```python
from build123d import *

# Parameters (mm, degrees)
SKETCH_1_W          = 35
SKETCH_1_H          = 3
EXTRUDE_1_DEPTH     = 3
SKETCH_2_R          = 1.75
CUT_EXTRUDE_1_DEPTH = 10
CHAMFER_1_SIZE      = 2


with BuildPart() as part:
    # Эскиз1 → Бобышка-Вытянуть1 (new body)
    with BuildSketch(Plane.XY):
        Polygon((-32.5, 50), (-32.5, -50), (32.5, -50), (32.5, 50), (17.5, 50), (17.5, 47), (-17.5, 47), (-17.5, 50), align=None)
        with Locations((0, 48.5)):
            Rectangle(SKETCH_1_W, SKETCH_1_H)
        with Locations((0, 51.5)):
            Rectangle(SKETCH_1_W, SKETCH_1_H)
    extrude(amount=EXTRUDE_1_DEPTH)

    # Эскиз2 → Вырез-Вытянуть1 (cut)
    with BuildSketch(Plane.XY.offset(3)):
        with Locations((-25.8, 27.95)):
            Circle(SKETCH_2_R)
        with Locations((-7, 27.95)):
            Circle(SKETCH_2_R)
        with Locations((7, 27.95)):
            Circle(SKETCH_2_R)
        with Locations((25.8, 27.95)):
            Circle(SKETCH_2_R)
        with Locations((-25.8, -27.95)):
            Circle(SKETCH_2_R)
        with Locations((-7, -27.95)):
            Circle(SKETCH_2_R)
        with Locations((7, -27.95)):
            Circle(SKETCH_2_R)
        with Locations((25.8, -27.95)):
            Circle(SKETCH_2_R)
    extrude(amount=-CUT_EXTRUDE_1_DEPTH, mode=Mode.SUBTRACT)

    # Фаска1
    chamfer_1_edges = [part.edges().sort_by_distance(p)[0] for p in [
        (-27.55, -27.95, 0),
        (24.05, 27.95, 0),
        (5.25, 27.95, 0),
        (-8.75, 27.95, 0),
        (-8.75, -27.95, 0),
        (5.25, -27.95, 0),
        (24.05, -27.95, 0),
        (-27.55, 27.95, 0),
    ]]
    chamfer(chamfer_1_edges, length=CHAMFER_1_SIZE)


solid = part.part
```
Design review of the part built by this model. Coordinates are the model's own, in mm. A direction names the side the tool comes from. Round coordinates to 2 decimals unless told otherwise and drop trailing zeros. Order: outer loops, then holes, each group sorted by start corner. A loop starts at its lowest first (then second) coordinate and runs counter-clockwise, first axis right, second up. Notation, with made-up numbers: (11.25, 17) - (32.25, 17) arc R9 cw to (32.25, 22) - close; hole circle Ø7 at (70, 70.5). An arc over 180 degrees is marked (long way). Return JSON: item names as keys, results as strings.
Q1. Consider section C-C on z = 0.55. Give the number of separate pieces and of enclosed holes in the cut face, plus the area to 3 significant figures.
Computed values:
{"separate pieces": "1", "enclosed holes": "8", "area": "6,350 mm2"}
Q2. Consider section D-D on x = -7. Write out the cut boundary in (y, z), plus the area to 3 significant figures.
Computed values:
{"outline": "(-50, 0) - (-31.7, 0) - (-29.7, 2) - (-29.7, 3) - (-50, 3) - close; (-26.2, 2) - (-24.2, 0) - (24.2, 0) - (26.2, 2) - (26.2, 3) - (-26.2, 3) - close; (29.7, 2) - (31.7, 0) - (53, 0) - (53, 3) - (29.7, 3) - close", "area": "280 mm2"}
Q3. Machinability: for faces 5 (the cylindrical face through (-26.028, 29.685, 2.507)), 6 (the flat face through (25, 50, 1)), which of the approach directions +Z, -Z, +X, -X, +Y, -Y give a long, thin tool a straight path to every point of the face, cutting with its end or side? Answer none if there is none.
Computed values:
{"face 5": "+Z, -Z", "face 6": "+Z, -Z, +X, +Y"}
Q4. Consider section B-B on y = 27.95. Write out the cut boundary in (x, z), plus the area to 3 significant figures.
Computed values:
{"outline": "(-32.5, 0) - (-29.55, 0) - (-27.55, 2) - (-27.55, 3) - (-32.5, 3) - close; (-24.05, 2) - (-22.05, 0) - (-10.75, 0) - (-8.75, 2) - (-8.75, 3) - (-24.05, 3) - close; (-5.25, 2) - (-3.25, 0) - (3.25, 0) - (5.25, 2) - (5.25, 3) - (-5.25, 3) - close; (8.75, 2) - (10.75, 0) - (22.05, 0) - (24.05, 2) - (24.05, 3) - (8.75, 3) - close; (27.55, 2) - (29.55, 0) - (32.5, 0) - (32.5, 3) - (27.55, 3) - close", "area": "137 mm2"}
Q5. Wall thickness on L1, parallel to Y at x = 25.8, z = 2.2; L2, parallel to Y at x = 7, z = 2.3; L3, parallel to X at y = 29, z = 0.65: over which ranges is each line inside the solid? List them lowest first. Write a range as [from, to].
Computed values:
{"L1": "y = [-50, -29.7], [-26.2, 26.2], [29.7, 50]", "L2": "y = [-50, -29.7], [-26.2, 26.2], [29.7, 53]", "L3": "x = [-32.5, -28.72], [-22.88, -9.92], [-4.08, 4.08], [9.92, 22.88], [28.72, 32.5]"}
Q6. Consider section A-A on x = -25.8. Write out the cut boundary in (y, z), plus the area to 3 significant figures.
Computed values:
{"outline": "(-50, 0) - (-31.7, 0) - (-29.7, 2) - (-29.7, 3) - (-50, 3) - close; (-26.2, 2) - (-24.2, 0) - (24.2, 0) - (26.2, 2) - (26.2, 3) - (-26.2, 3) - close; (29.7, 2) - (31.7, 0) - (50, 0) - (50, 3) - (29.7, 3) - close", "area": "271 mm2"}
Q7. For pin 1 Ø1.5 at (x, z) = (-21.5, 1.5) entering from +Y; pin 2 Ø4 at (x, y) = (-25.8, -27.95) entering from +Z; pin 3 Ø1.5 at (y, z) = (52, 2) entering from +X; pin 4 Ø3 at (x, y) = (-7, 27.95) entering from -Z, all flat-tipped, find the tip position at first contact; note any pin that passes through.
Computed values:
{"pin 1": "stops at y = 50", "pin 2": "stops at z = 3", "pin 3": "stops at x = 17.5", "pin 4": "passes through"}
Q8. The part is to be moulded in two halves that separate along X. For faces 1 (the flat face through (17.5, 51, 1)), 2 (the flat face through (-17.5, 51, 1)), 3 (the cylindrical face through (6.772, -26.215, 2.507)), 4 (the flat face through (0, 2, 0)), say which applies: pulls with the +X half, pulls with the -X half, needs draft (parallel to the pull), parting line crosses it, or undercut.
Computed values:
{"face 1": "pulls with the +X half", "face 2": "pulls with the -X half", "face 3": "undercut", "face 4": "needs draft"}
